```python
from build123d import *

# Parameters (mm, degrees)
SKETCH1_R           = 1.6
SKETCH1_W           = 15
SKETCH1_H           = 7
BOSS_EXTRUDE1_DEPTH = 2
FILLET1_R           = 5


with BuildPart() as part:
    # Sketch1 → Boss-Extrude1 (new body)
    with BuildSketch(Plane(origin=(0, 0, 0), x_dir=(1, 0, 0), z_dir=(0, 1, 0))):
        Polygon((62.361868445, 25.831131685), (62.361868445, -25.831131685), (25.831131685, -62.361868445), (-25.831131685, -62.361868445), (-62.361868445, -25.831131685), (-62.361868445, 25.831131685), (-25.831131685, 62.361868445), (25.831131685, 62.361868445), align=None)
        with Locations(Location((10, -42.5, 0), (0, 0, 270))):
            Circle(SKETCH1_R, mode=Mode.SUBTRACT)
        with Locations(Location((-10, -42.5, 0), (0, 0, 270))):
            Circle(SKETCH1_R, mode=Mode.SUBTRACT)
        with Locations(Location((-10, 42.5, 0), (0, 0, 270))):
            Circle(SKETCH1_R, mode=Mode.SUBTRACT)
        with Locations(Location((10, 42.5, 0), (0, 0, 270))):
            Circle(SKETCH1_R, mode=Mode.SUBTRACT)
        with BuildLine():
            Line((12.5, -55), (-12.5, -55))
            ThreePointArc((-12.5, -55), (-17.5, -50), (-12.5, -45))
            Line((-12.5, -45), (12.5, -45))
            ThreePointArc((12.5, -45), (17.5, -50), (12.5, -55))
        make_face(mode=Mode.SUBTRACT)
        with BuildLine():
            Line((12.5, 55), (-12.5, 55))
            ThreePointArc((-12.5, 55), (-17.5, 50), (-12.5, 45))
            Line((-12.5, 45), (12.5, 45))
            ThreePointArc((12.5, 45), (17.5, 50), (12.5, 55))
        make_face(mode=Mode.SUBTRACT)
        with Locations((0, -18.5)):
            Rectangle(SKETCH1_W, SKETCH1_H, mode=Mode.SUBTRACT)
        with Locations((0, 18.5)):
            Rectangle(SKETCH1_W, SKETCH1_H, mode=Mode.SUBTRACT)
    extrude(amount=BOSS_EXTRUDE1_DEPTH)

    # Fillet1
    fillet1_edges = [part.edges().sort_by_distance(p)[0] for p in [
        (-62.361868445, 1, -25.831131685),
        (-25.831131685, 1, -62.361868445),
        (25.831131685, 1, -62.361868445),
        (62.361868445, 1, -25.831131685),
        (62.361868445, 1, 25.831131685),
        (25.831131685, 1, 62.361868445),
        (-25.831131685, 1, 62.361868445),
        (-62.361868445, 1, 25.831131685),
    ]]
    fillet(fillet1_edges, radius=FILLET1_R)


solid = part.part
```
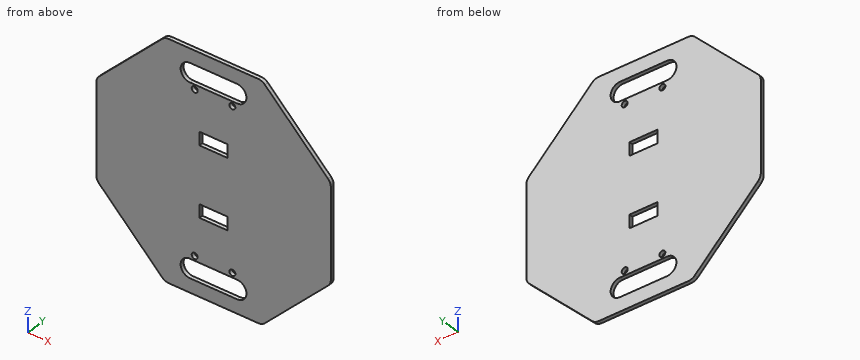
Here's how the part is built. I have some questions about the finished solid (model axes, mm). Round coordinates to 2 decimals unless told otherwise and drop trailing zeros. Write each loop counter-clockwise with the first axis right and the second up, starting at its lowest first coordinate (ties: lowest second). Pieces come first, ordered by that corner, then holes.
Q1. If we section it at D-D on z = -35.5: Write out the boundary of the cut face in (x, y).
Q2. Please list where these lines run through material, in increasing order: probe 1 along Z at (x, y) = (2, 1.4); probe 2 along X at (y, z) = (0.8, -42.5); probe 3 along Z at (x, y) = (46, 0.2).
Q3. If we section it at B-B on z = 42.5: Write out the boundary of the cut face in (x, y).
Q4. If we section it at A-A on x = 10: Write out the boundary of the cut face in (y, z), plus the area to 3 significant figures.
Q5. If we section it at C-C on y = 0.65: Give the number of separate pieces and of enclosed holes in the cut face, plus the area to 3 significant figures.
Answer below:
1. outline: (-52.69, 0) - (52.69, 0) - (52.69, 2) - (-52.69, 2) - close
2. probe 1: z = -62.36 to -55, -45 to -22, -15 to 15, 22 to 45, 55 to 62.36
2. probe 2: x = -45.69 to -11.6, -8.4 to 8.4, 11.6 to 45.69
2. probe 3: z = -42.19 to 42.19
3. outline: (-45.69, 0) - (-11.6, 0) - (-11.6, 2) - (-45.69, 2) - close; (-8.4, 0) - (8.4, 0) - (8.4, 2) - (-8.4, 2) - close; (11.6, 0) - (45.69, 0) - (45.69, 2) - (11.6, 2) - close
4. outline: (0, -62.36) - (2, -62.36) - (2, -55) - (0, -55) - close; (0, -45) - (2, -45) - (2, -44.1) - (0, -44.1) - close; (0, -40.9) - (2, -40.9) - (2, 40.9) - (0, 40.9) - close; (0, 44.1) - (2, 44.1) - (2, 45) - (0, 45) - close; (0, 55) - (2, 55) - (2, 62.36) - (0, 62.36) - close
4. area: 197 mm2
5. separate pieces: 1
5. enclosed holes: 8
5. area: 12,000 mm2
